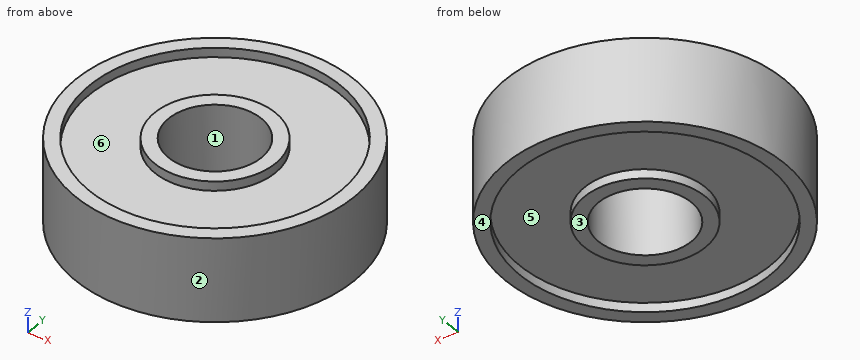
Autodesk Inventor part; units mm, degrees
ref_plane "YZ Plane" through (0, 0, 0) normal (1, 0, 0) x (0, 1, 0)
ref_plane "XZ Plane" through (0, 0, 0) normal (0, 1, 0) x (-1, 0, 0)
ref_plane "XY Plane" through (0, 0, 0) normal (0, 0, 1) x (1, 0, 0)
sketch "Szkic1" plane through (0, 0, 0) normal (0, 0, 1) x (1, 0, 0)
  circle A0 centre (0, 0) radius 5
  circle A1 centre (0, 0) radius 15
  dimension "d0" = 10
  dimension "d1" = 30
extrude "Wyciągnięcie proste1" add sketch "Szkic1" along normal blind 9
sketch "Szkic2" plane through (0, 0, 9) normal (0, 0, 1) x (1, 0, 0)
  circle A0 centre (0, 0) radius 5
  circle A1 centre (0, 0) radius 15
  circle A2 centre (0, 0) radius 6.5
  circle A3 centre (0, 0) radius 13.5
  dimension "d4" = 13
  dimension "d5" = 27
extrude "Wyciągnięcie proste2" cut sketch "Szkic2" against normal blind 1 contours A3
sketch "Szkic3" plane through (0, 0, 0) normal (0, 0, -1) x (-1, 0, 0)
  circle A0 centre (0, 0) radius 6.5
  circle A1 centre (0, 0) radius 13.5
  dimension "d8" = 13
  dimension "d9" = 27
extrude "Wyciągnięcie proste3" cut sketch "Szkic3" against normal blind 1
properties part number "Łożysko kulowe jednorzędowe 6200 2RS"
Model file for the job. Use its own axes, mm. Face numbers are marked on the shaded views. A direction names the side the tool comes from. Round coordinates to 2 decimals unless told otherwise and drop trailing zeros. Write each loop counter-clockwise with the first axis right and the second up, starting at its lowest first coordinate (ties: lowest second). Pieces come first, ordered by that corner, then holes. Notation, with made-up numbers: (-15.75, 22.25) -> (-0.75, 22.25) arc R20 cw to (-0.75, 57.25) -> close; hole circle Ø11 at (83.25, 70). An arc over 180 degrees is marked (long way). Answer as CSV lines item,"result".
1. Tool access for the marked faces 4, 5 and 6: list every direction of +Z, -Z, +X, -X, +Y, -Y with a clear straight run to the whole face (end or side of a thin tool).
Resolved:
face 4,"-Z, +X, -X, +Y, -Y"
face 5,"-Z"
face 6,"+Z"
2. Slice it at D-D, the plane y = -11.5. List the corners of the cut face in (x, z).
Resolved:
outline,"(-9.63, 0) -> (-7.07, 0) -> (-7.07, 1) -> (7.07, 1) -> (7.07, 0) -> (9.63, 0) -> (9.63, 9) -> (7.07, 9) -> (7.07, 8) -> (-7.07, 8) -> (-7.07, 9) -> (-9.63, 9) -> close"
3. Pin check, flat tips, straight feed: pin 1 Ø5 at (y, z) = (-5.5, 2) entering from -X; pin 2 Ø1 at (y, z) = (4, 4) entering from +X; pin 3 Ø2 at (y, z) = (8, 5.5) entering from -X. Stop position of each tip, or through.
Resolved:
pin 1,"x = -14.7"
pin 2,"x = 14.59"
pin 3,"x = -13.27"
4. Slice it at C-C, the plane z = 3.25. List the corners of the cut face in (x, y).
Resolved:
outline,"circle Ø30 at (0, 0); hole circle Ø10 at (0, 0)"
5. Mould opens along Y. For the marked faces 1, 2 and 3 say: +Y half, -Y half, draft (parallel to the pull), parting line (faces both ways), or undercut.
Resolved:
face 1,"undercut"
face 2,"parting line"
face 3,"draft"
6. Slice it at A-A, the plane x = 0. List the corners of the cut face in (y, z).
Resolved:
outline,"(-15, 0) -> (-13.5, 0) -> (-13.5, 1) -> (-6.5, 1) -> (-6.5, 0) -> (-5, 0) -> (-5, 9) -> (-6.5, 9) -> (-6.5, 8) -> (-13.5, 8) -> (-13.5, 9) -> (-15, 9) -> close; (5, 0) -> (6.5, 0) -> (6.5, 1) -> (13.5, 1) -> (13.5, 0) -> (15, 0) -> (15, 9) -> (13.5, 9) -> (13.5, 8) -> (6.5, 8) -> (6.5, 9) -> (5, 9) -> close"
7. Drill centre lines: line 1 (Y direction, x = 0, z = 8.4); line 2 (Y direction, x = -0.25, z = 4.5); line 3 (X direction, y = 2.5, z = 4.25). Where is each one in solid material? Low to high.
Resolved:
line 1,"-15 to -13.5, -6.5 to -5, 5 to 6.5, 13.5 to 15"
line 2,"-15 to -4.99, 4.99 to 15"
line 3,"-14.79 to -4.33, 4.33 to 14.79"
